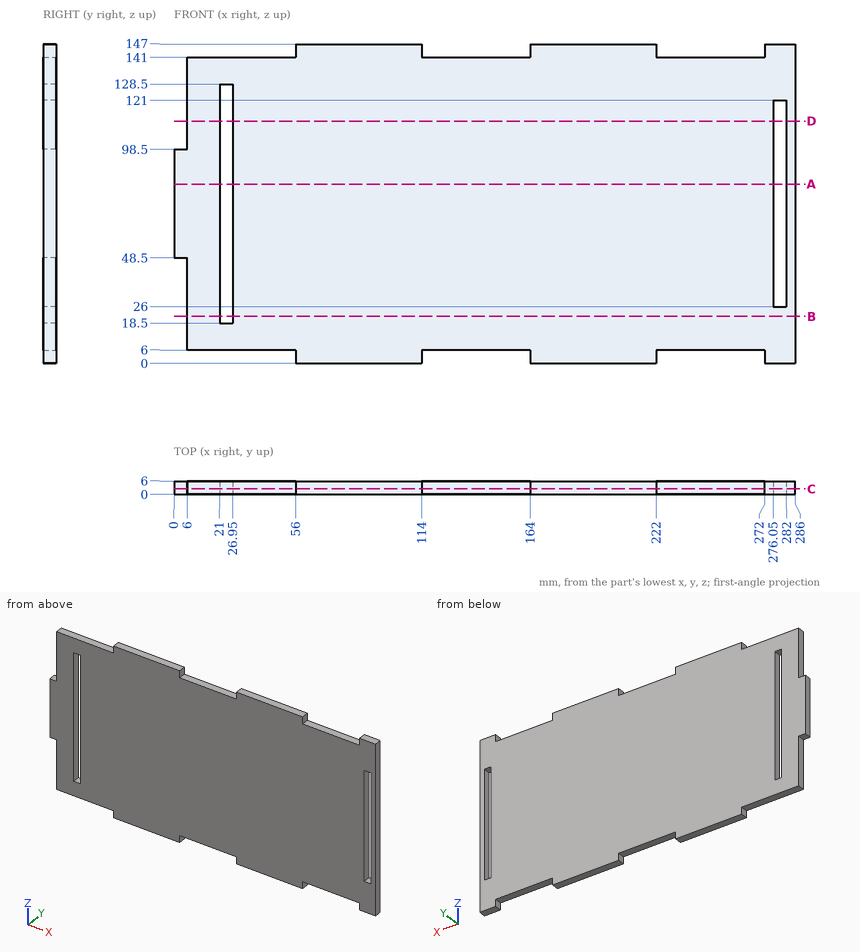
Study the drawing (mm; zero at the part's minimum x, y, z) and answer. Coordinates: 2 decimals unless noted, no trailing zeros. Write each loop counter-clockwise with the first axis right and the second up, starting at its lowest first coordinate (ties: lowest second). Pieces come first, ordered by that corner, then holes.
Q1. Find the intervals of material crossed by line 1 (X direction, y = 3.65, z = 55); line 2 (X direction, y = 5.65, z = 42.5); line 3 (X direction, y = 5.7, z = 23), in increasing order.
Q2. A cutting plane is placed at C-C, the plane y = 2.5. State how many separate pieces and enclosed holes the cut face has, then the cut area to 3 significant figures.
Q3. A cutting plane is placed at B-B, the plane z = 21.5. Give the vertices of the cut face in (x, y).
Q4. A cutting plane is placed at A-A, the plane z = 82.5. Give the vertices of the cut face in (x, y).
Q5. A cutting plane is placed at D-D, the plane z = 111.5. Give the vertices of the cut face in (x, y), then the cut area to 3 significant figures.
Q6. This flat-tipped pin is pushed along its axis until it touches: pin 1 Ø3 at (x, y) = (132, 3.5) entering from +Z. Where does it stop, or does it pass through?
Findings below:
1. line 1: x = 0 to 21, 26.95 to 276.05, 282 to 286
1. line 2: x = 6 to 21, 26.95 to 276.05, 282 to 286
1. line 3: x = 6 to 21, 26.95 to 286
2. separate pieces: 1
2. enclosed holes: 2
2. area: 38,400 mm2
3. outline: (6, 0) - (21, 0) - (21, 6) - (6, 6) - close; (26.95, 0) - (286, 0) - (286, 6) - (26.95, 6) - close
4. outline: (0, 0) - (21, 0) - (21, 6) - (0, 6) - close; (26.95, 0) - (276.05, 0) - (276.05, 6) - (26.95, 6) - close; (282, 0) - (286, 0) - (286, 6) - (282, 6) - close
5. outline: (6, 0) - (21, 0) - (21, 6) - (6, 6) - close; (26.95, 0) - (276.05, 0) - (276.05, 6) - (26.95, 6) - close; (282, 0) - (286, 0) - (286, 6) - (282, 6) - close
5. area: 1,610 mm2
6. pin 1: stops at z = 141
